Input: part model. Units: mm. Frame: model coordinates. A direction names the side the tool comes from. Round coordinates to 2 decimals unless told otherwise and drop trailing zeros. Order: outer loops, then holes, each group sorted by start corner. A loop starts at its lowest first (then second) coordinate and runs counter-clockwise, first axis right, second up.
Item 1: Reachability of faces 5 (the flat face through (-3, 0, 0)), 6 (the flat face through (-2, -4, -2.6)), 7 (the cylindrical face through (2.192, 2.092, -4.214)) from +Z, -Z, +X, -X, +Y, -Y: full face, straight path, thin tool, end or side. Return the list, or none.
Item 2: First-contact query: pin 1 (1 mm diameter, centred on x = 4, y = -3.5, fed in from +Z); pin 2 (1 mm diameter, centred on x = -2, y = -4.5, fed in from +Z); pin 3 (4 mm diameter, centred on x = -1, y = -2.5, fed in from +Z); pin 4 (3 mm diameter, centred on x = 2.5, z = -2, fed in from +Y). Flat tips, straight axial feed; report the tip coordinate or a pass-through.
Item 3: Mould query, pull axis Z, two halves, no side actions, for faces 1 (the flat face through (-4.1, -2.1, 0)), 2 (the cylindrical face through (2.097, -3.317, 3.288)), 3 (the flat face through (3.3, -3.5, -1.1)), 4 (the cylindrical face through (-2.46, -4.19, -1.886)). Classes: released by +Z, released by -Z, zero draft, split by the parting line, or undercut.
Item 4: Cut plane C-C on z = 0. Output: boundary loops of the cut face in (x, y).
Item 5: Cut plane A-A on x = 0. Output: boundary loops of the cut face in (y, z), then the cut area to 3 significant figures.
Item 6: Line query: L1, parallel to Z at x = 0, y = 2; L2, parallel to Z at x = 0, y = -5.5; L3, parallel to X at y = -5.5, z = 0. Output: solid intervals per line, ascending.
Item 7: Cut plane B-B on y = -4.75. Give the number of separate pieces and of enclosed holes in the cut face, then the cut area to 3 significant figures.
```python
from build123d import *

# Parameters (mm, degrees)
SKETCH2_W               = 0.5
SKETCH2_H               = 7
CUT_EXTRUDE1_DEPTH      = 5.75
CUT_EXTRUDE1_DEPTH_BACK = 5.75
BOSS_EXTRUDE1_DEPTH     = 1.2
CHAMFER1_SIZE           = 0.5


with BuildPart() as part:
    # Sketch1 → Revolve1 (revolve)
    with BuildSketch(Plane.XY):
        Polygon((2.6, 0), (2.6, 4), (4.75, 2.7), (4.75, 1.5), (3.9, 1.5), (3.9, -8.5), (3.1, -8.5), (3.1, 0), align=None)
    revolve(axis=Axis((0, 42.244045278, 0), (0, -1, 0)))

    # Sketch2 → Cut-Extrude1 (cut, two sides)
    with BuildSketch(Plane(origin=(0, 0, 0), x_dir=(0, 0, -1), z_dir=(1, 0, 0))) as cut_extrude1_sk:
        Polygon((0.6, -7), (1.1, -7), (1.1, 0), (-1.1, 0), (-1.1, -7), (-0.6, -7), (-0.6, -0.5), (0.6, -0.5), align=None)
        with Locations((-2.35, -3.5)):
            Rectangle(SKETCH2_W, SKETCH2_H)
        with Locations((2.35, -3.5)):
            Rectangle(SKETCH2_W, SKETCH2_H)
    extrude(amount=CUT_EXTRUDE1_DEPTH, mode=Mode.SUBTRACT)
    extrude(cut_extrude1_sk.sketch, amount=-CUT_EXTRUDE1_DEPTH_BACK, mode=Mode.SUBTRACT)

    # Sketch3 → Boss-Extrude1 (add)
    with BuildSketch(Plane.XY.offset(0.6)):
        Polygon((3.853569774, -0.5), (4.353569774, -3.75), (3.853569774, -7), align=None)
    boss_extrude1 = extrude(amount=-BOSS_EXTRUDE1_DEPTH)

    # Mirror1: Boss-Extrude1 across plane
    add(boss_extrude1.mirror(Plane(origin=(0, 0, 0), x_dir=(0, 0, 1), z_dir=(1, 0, 0))))

    # Chamfer1
    chamfer1_edges = [part.edges().sort_by_distance(p)[0] for p in [
        (-3.9, -8.5, 0),
    ]]
    chamfer(chamfer1_edges, length=CHAMFER1_SIZE)


solid = part.part
```
From the geometry:
1. face 5: none
1. face 6: +X, -X
1. face 7: +Y, -Y
2. pin 1: stops at z = 1.72
2. pin 2: stops at z = 3.6
2. pin 3: stops at z = 3.9
2. pin 4: stops at y = 4
3. face 1: zero draft
3. face 2: split by the parting line
3. face 3: undercut
3. face 4: undercut
4. outline: (-4.75, 1.5) - (-3.9, 1.5) - (-3.9, 0) - (-2.6, 0) - (-2.6, 4) - (-4.75, 2.7) - close; (-4.35, -3.75) - (-3.9, -6.7) - (-3.9, -8) - (-3.4, -8.5) - (-3.1, -8.5) - (-3.1, -0.5) - (-3.9, -0.5) - (-3.9, -0.8) - close; (2.6, 0) - (3.9, 0) - (3.9, 1.5) - (4.75, 1.5) - (4.75, 2.7) - (2.6, 4) - close; (3.1, -8.5) - (3.4, -8.5) - (3.9, -8) - (3.9, -6.7) - (4.35, -3.75) - (3.9, -0.8) - (3.9, -0.5) - (3.1, -0.5) - close
5. outline: (-8.5, -3.4) - (-8, -3.9) - (1.5, -3.9) - (1.5, -4.75) - (2.7, -4.75) - (4, -2.6) - (0, -2.6) - (0, -3.1) - (-8.5, -3.1) - close; (-8.5, 3.1) - (0, 3.1) - (0, 2.6) - (4, 2.6) - (2.7, 4.75) - (1.5, 4.75) - (1.5, 3.9) - (-8, 3.9) - (-8.5, 3.4) - close
5. area: 25.2 mm2
6. L1: z = -4.75 to -2.6, 2.6 to 4.75
6. L2: z = -3.9 to -3.1, 3.1 to 3.9
6. L3: x = -4.08 to -3.1, 3.1 to 4.08
7. separate pieces: 8
7. enclosed holes: 0
7. area: 14.5 mm2
